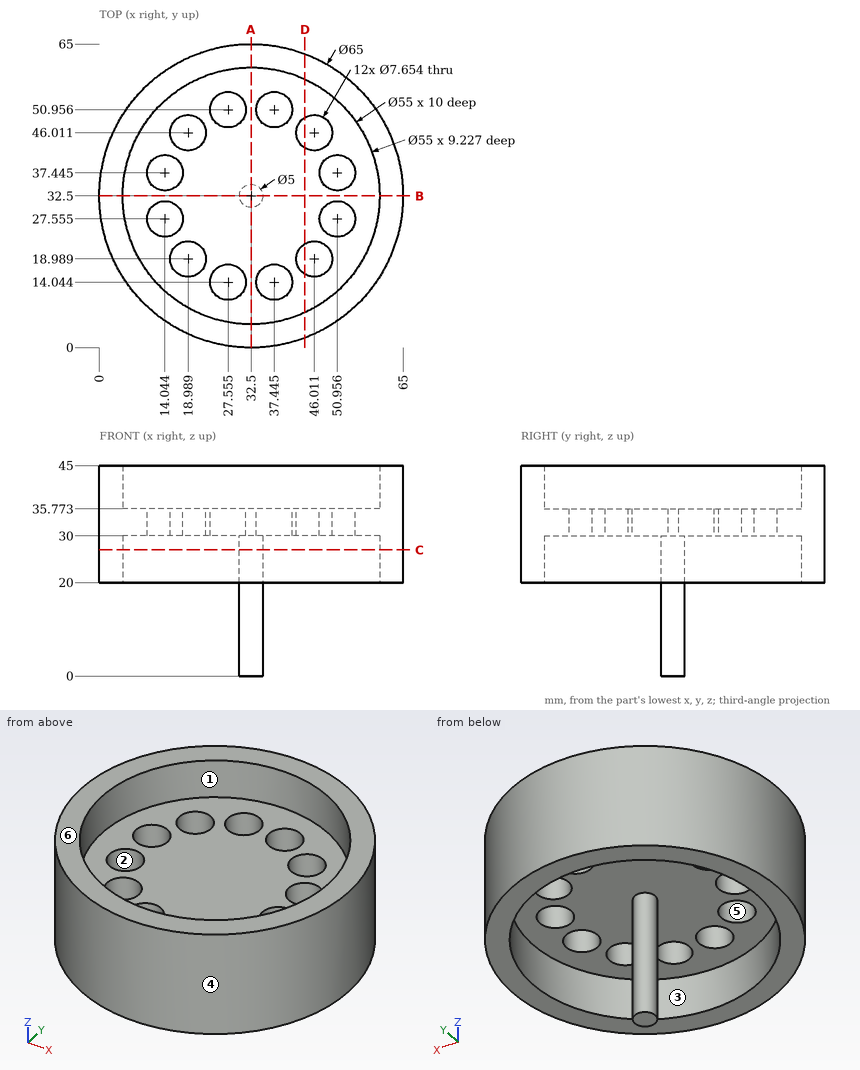
The figure shows three views and two pictorial views of one solid part (mm, origin at its lowest corner). Answer the questions. A direction names the side the tool comes from. Coordinates: 2 decimals unless noted, no trailing zeros. Write each loop counter-clockwise with the first axis right and the second up, starting at its lowest first coordinate (ties: lowest second). Pieces come first, ordered by that corner, then holes. Notation, with made-up numbers: M -7,43 L 3,43 A17 cw 3,73 Z; hole C 86,57.5 d7. An arc over 180 degrees is marked long. Answer as CSV lines item,"result". Start each with the question number.
Item 1: Consider L1, parallel to Y at x = 32.5, z = 25; L2, parallel to Z at x = 32.5, y = 14; L3, parallel to X at y = 51, z = 38.5 (1 decimal). Determine where each line is inside the solid, lowest interval first.
Item 2: A tool of negligible diameter and unlimited length cuts with its end or side. For the marked faces 1, 2 and 3, from which of +Z, -Z, +X, -X, +Y, -Y can it reach the whole face along a straight path? Write none if from no direction.
Item 3: Section A-A on x = 32.5 is taken. Write down the section's boundary in (y, z).
Item 4: Flat-ended cylindrical pins translate along their axes: P1, Ø3, axis at x = 29.5, z = 25, coming from the +Y side (1 decimal); P2, Ø5, axis at y = 45, z = 20, coming from the -X side; P3, Ø1.5, axis at x = 44, z = 36, coming from the -Y side; P4, Ø4.5, axis at x = 27.55, y = 50.96, coming from the -Z side. Find the tip coordinate at first contact, or state that the pin passes through.
Item 5: Section C-C on z = 27 is taken. Write down the section's boundary in (x, y).
Item 6: Determine the mould class of the marked faces 4, 5 and 6 for opening direction Y: released by +Y, released by -Y, zero draft, split by the parting line, or undercut.
Item 7: Section D-D on x = 44 is taken. Write down the section's boundary in (y, z), and give its area (3 significant figures).
Checks:
1,L1,"y = 0 to 5, 30 to 35, 60 to 65"
1,L2,"z = 30 to 35.77"
1,L3,"x = 5.8 to 12.2, 52.8 to 59.2"
2,face 1,"+Z"
2,face 2,"+Z, -Z"
2,face 3,"-Z"
3,outline,"M 0,20 L 5,20 L 5,30 L 30,30 L 30,0 L 35,0 L 35,30 L 60,30 L 60,20 L 65,20 L 65,45 L 60,45 L 60,35.77 L 5,35.77 L 5,45 L 0,45 Z"
4,P1,"stops at y = 65"
4,P2,"stops at x = 1.58"
4,P3,"stops at y = 1.83"
4,P4,"passes through"
5,outline,"C 32.5,32.5 d65; C 32.5,32.5 d5; hole C 32.5,32.5 d55"
6,face 4,"split by the parting line"
6,face 5,"undercut"
6,face 6,"zero draft"
7,outline,"M 2.1,20 L 7.52,20 L 7.52,30 L 15.73,30 L 15.73,35.77 L 7.52,35.77 L 7.52,45 L 2.1,45 Z; M 22.25,30 L 42.75,30 L 42.75,35.77 L 22.25,35.77 Z; M 49.27,30 L 57.48,30 L 57.48,20 L 62.9,20 L 62.9,45 L 57.48,45 L 57.48,35.77 L 49.27,35.77 Z"
7,area,"484 mm²"
